Could you check a few things on this model? Use its own coordinates, in mm. A direction names the side the tool comes from. Round coordinates to 2 decimals unless told otherwise and drop trailing zeros. Loops run counter-clockwise (first coordinate to the right, second up) from the corner with the lowest first, then second, coordinate; pieces in that order, holes last. Notation, with made-up numbers: (0, 63.25) - (52, 63.25) arc R17 cw to (52, 68.25) - close; hole circle Ø11 at (-35, -8.75). An arc over 180 degrees is marked (long way). Put each result on its own line as item: value. Start each with the question number.
from build123d import *

# Parameters (mm, degrees)
F0_W     = 50.8
F0_H     = 25.4
F1_DEPTH = 50.8
F2_SIZE  = 6.35
F3_SIZE  = 6.35
F4_T     = -2.54


with BuildPart() as f1:
    # F0 (on Front) → F1 (new body)
    with BuildSketch(Plane.XZ):
        with Locations((-55.30939, -62.134533)):
            Rectangle(F0_W, F0_H)
    extrude(amount=F1_DEPTH)

    # F2
    f2_edges = [f1.edges().sort_by_distance(p)[0] for p in [
        (-29.90939, -25.4, -74.834533),
    ]]
    chamfer(f2_edges, length=F2_SIZE)

    # F3
    f3_edges = [f1.edges().sort_by_distance(p)[0] for p in [
        (-80.70939, -25.4, -74.834533),
    ]]
    chamfer(f3_edges, length=F3_SIZE)

    # F4
    f4_openings = [f1.faces().sort_by_distance(p)[0] for p in [
        (-55.30939, -25.4, -49.434533),
    ]]
    offset(amount=F4_T, openings=f4_openings)


solid = f1.part
Item 1: Suppose I cut it at B-B, the plane y = -38.5. List the corners of the cut face in (x, z) for me.
Item 2: Thinking about a two-plate mould opening in Y: for faces 3 (the face through (-56, 0, -62)), 4 (the face through (-56, -25, -72.295)), 5 (the face through (-29.909, -25, -59)), which applies, released by +Y, released by -Y, zero draft, split by the parting line, or undercut?
Item 3: I need wall thicknesses on line 1 (X direction, y = -21, z = -57.75); line 2 (Y direction, x = -60, z = -71.25); line 3 (Z direction, x = -60, y = -10.5). Which ranges of each line are inside material? Lowest first, please. Write a range as from..to.
Item 4: Suppose I cut it at C-C, the plane x = -48.5. List the corners of the cut face in (y, z) for me.
Item 5: On a 3-axis mill with a long thin cutter (end or side, diameter ignored), from which of +Z, -Z, +X, -X, +Y, -Y can I reach the whole of each face in a straight line? I mean faces 1 (the face through (-33.04, -25.044, -71.615)), 2 (the face through (-34.846, -25.08, -69.829)). Say none if no direction works.
Item 6: Will this pin go through, and if not, where does the flat tip stop? P1, Ø3, axis at x = -75.5, y = -43, coming from the -Z side.
Item 7: Suppose I cut it at D-D, the plane z = -69.75. List the corners of the cut face in (x, y) for me, then the cut area to 3 significant figures.
Item 8: Suppose I cut it at A-A, the plane z = -55. List the corners of the cut face in (x, y) for me.
Numbers:
1. outline: (-80.71, -68.48) - (-74.36, -74.83) - (-36.26, -74.83) - (-29.91, -68.48) - (-29.91, -49.43) - (-32.45, -49.43) - (-32.45, -67.43) - (-37.31, -72.29) - (-73.31, -72.29) - (-78.17, -67.43) - (-78.17, -49.43) - (-80.71, -49.43) - close
2. face 3: released by +Y
2. face 4: undercut
2. face 5: zero draft
3. line 1: -80.71..-78.17, -32.45..-29.91
3. line 2: -50.8..-48.26, -2.54..0
3. line 3: -74.83..-72.29
4. outline: (-50.8, -74.83) - (0, -74.83) - (0, -49.43) - (-2.54, -49.43) - (-2.54, -72.29) - (-48.26, -72.29) - (-48.26, -49.43) - (-50.8, -49.43) - close
5. face 1: -Z, +X, +Y, -Y
5. face 2: +Z
6. P1: z = -74.83
7. outline: (-79.44, -50.8) - (-31.17, -50.8) - (-31.17, 0) - (-79.44, 0) - close; hole (-75.85, -48.26) - (-34.77, -48.26) - (-34.77, -2.54) - (-75.85, -2.54) - close
7. area: 574 mm^2
8. outline: (-80.71, -50.8) - (-29.91, -50.8) - (-29.91, 0) - (-80.71, 0) - close; hole (-78.17, -48.26) - (-32.45, -48.26) - (-32.45, -2.54) - (-78.17, -2.54) - close
